Read the model definition and answer for the solid it produces. Units are mm, in the model's axes. Face numbers are marked on the shaded views. A direction names the side the tool comes from. Round coordinates to 2 decimals unless told otherwise and drop trailing zeros. Write each loop counter-clockwise with the first axis right and the second up, starting at its lowest first coordinate (ties: lowest second). Pieces come first, ordered by that corner, then holes. Notation, with made-up numbers: (52.25, 8) -> (59.25, 8) arc R19 cw to (59.25, 28) -> close; hole circle Ø1 at (-40, 52). An arc over 180 degrees is marked (long way). Return JSON: item names as keys, results as strings.
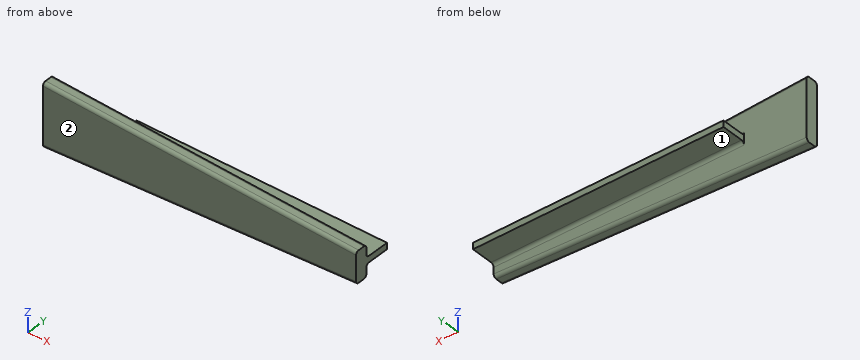
from build123d import *

# Parameters (mm, degrees)
BOSS_EXTRUDE1_DEPTH = 2
SKETCH2_W           = 40
SKETCH2_H           = 1
BOSS_EXTRUDE2_DEPTH = 4
FILLET1_R           = 0.5


with BuildPart() as part:
    # Sketch1 → Boss-Extrude1 (new body)
    with BuildSketch(Plane(origin=(0, 0, 0), x_dir=(1, 0, 0), z_dir=(0, 1, 0))):
        Polygon((0, -5), (0, 5), (50, 2.5), (50, -2.5), align=None)
    extrude(amount=BOSS_EXTRUDE1_DEPTH)

    # Sketch2 → Boss-Extrude2 (add)
    with BuildSketch(Plane(origin=(0, 2, 0), x_dir=(1, 0, 0), z_dir=(0, 1, 0))):
        with Locations((30, 0)):
            Rectangle(SKETCH2_W, SKETCH2_H)
    extrude(amount=BOSS_EXTRUDE2_DEPTH)

    # Fillet1
    fillet1_edges = [part.edges().sort_by_distance(p)[0] for p in [
        (25, 2, 3.75),
        (30, 2, -0.5),
        (30, 2, 0.5),
        (25, 2, -3.75),
        (25, 0, 3.75),
        (25, 0, -3.75),
    ]]
    fillet(fillet1_edges, radius=FILLET1_R)


solid = part.part
Item 1: A tool of negligible diameter and unlimited length cuts with its end or side. For the marked faces 1 and 2, from which of +Z, -Z, +X, -X, +Y, -Y can it reach the whole face along a straight path? Write none if from no direction.
Worked answers:
{"face 1": "-Z, +X, -X, +Y", "face 2": "+Z, -Z, +X, -X, -Y"}
Item 2: Section A-A (y = 3.45) is taken. Give the vertices of the cut face in (x, z).
Worked answers:
{"outline": "(10, -0.5) -> (50, -0.5) -> (50, 0.5) -> (10, 0.5) -> close"}
Item 3: Straight lines are drawn through the part: L1, parallel to Y at x = 47, z = 2; L2, parallel to Z at x = 44.5, y = 5; L3, parallel to Z at x = 9, y = 1.3. For each, find the intervals that lie inside material, in ascending order. Write a range as [from, to].
Worked answers:
{"L1": "y = [0, 2]", "L2": "z = [-0.5, 0.5]", "L3": "z = [-4.55, 4.55]"}
Item 4: Flat-ended cylindrical pins translate along their axes: pin 1 (3 mm diameter, centred on x = 25, y = 4.5, fed in from -Z); pin 2 (2 mm diameter, centred on x = 30, z = 2.5, fed in from +Y); pin 3 (1.5 mm diameter, centred on y = 4, z = 1, fed in from -X). Find the tip coordinate at first contact, or state that the pin passes through.
Worked answers:
{"pin 1": "stops at z = -0.5", "pin 2": "stops at y = 2", "pin 3": "stops at x = 10"}
Item 5: Section B-B (z = -1.5) is taken. Give the vertices of the cut face in (x, y), then the cut area to 3 significant figures.
Worked answers:
{"outline": "(0, 0) -> (50, 0) -> (50, 2) -> (0, 2) -> close", "area": "100 mm2"}
